from build123d import *

# Parameters (mm, degrees)
F1_DEPTH = 63.5
F0_W     = 25.4
F0_H     = 19.05
F2_DEPTH = 25.4
F3_DEPTH = 7.9375
F4_R     = 6.35


with BuildPart() as f1:
    # F0 (on Front) → F1 (new body, symmetric)
    with BuildSketch(Plane.XZ):
        Polygon((41.275, -9.525), (41.275, 9.525), (22.225, 9.525), (-41.275, 9.525), (-41.275, -9.525), align=None)
    extrude(amount=F1_DEPTH, both=True)

    # F0 (on Front) → F2 (join, symmetric)
    with BuildSketch(Plane.XZ):
        with BuildLine():
            Line((22.225, 9.525), (41.275, 9.525))
            Line((41.275, 9.525), (41.275, 27.0002))
            ThreePointArc((41.275, 27.0002), (45.9246798487, 38.2255201513), (57.15, 42.8752))
            Line((57.15, 42.8752), (60.325, 42.8752))
            Line((60.325, 42.8752), (60.325, 61.9252))
            Line((60.325, 61.9252), (57.15, 61.9252))
            add(Edge.make_bspline(
                [(54.22326899, 61.8023532465), (55.2121587279, 61.8549706116), (56.1881793337, 61.8959521575), (57.15, 61.9252)],
                knots=[108.6829517829, 108.6829517829, 108.6829517829, 108.6829517829, 111.5045361635, 111.5045361635, 111.5045361635, 111.5045361635], degree=3))
            ThreePointArc((54.22326899, 61.8023532465), (31.440354869, 50.6385115352), (22.225, 27.0002))
            Line((22.225, 27.0002), (22.225, 9.525))
        make_face()
        with Locations((73.025, 52.4002)):
            Rectangle(F0_W, F0_H)
    extrude(amount=F2_DEPTH, both=True)

    # F0 (on Front) → F3 (join, symmetric)
    with BuildSketch(Plane.XZ):
        with BuildLine():
            Line((-41.275, 9.525), (22.225, 9.525))
            Line((22.225, 9.525), (22.225, 27.0002))
            ThreePointArc((22.225, 27.0002), (31.440354869, 50.6385115352), (54.22326899, 61.8023532465))
            add(Edge.make_bspline(
                [(-41.275, 9.525), (-41.0511784846, 40.4851844974), (16.1328058977, 59.7756158605), (54.22326899, 61.8023532465)],
                knots=[0, 0, 0, 0, 108.6829517829, 108.6829517829, 108.6829517829, 108.6829517829], degree=3))
        make_face()
    extrude(amount=F3_DEPTH, both=True)

    # F4
    f4_edges = [f1.edges().sort_by_distance(p)[0] for p in [
        (41.275, -63.5, 0),
        (-41.275, -63.5, 0),
        (-41.275, 63.5, 0),
        (41.275, 63.5, 0),
    ]]
    fillet(f4_edges, radius=F4_R)


solid = f1.part
Geometry check sheet. Reference: the model listing, model coordinates, mm. A direction names the side the tool comes from. Give positions to 0.01 mm unless a question says otherwise; leave off trailing zeros. Loops run counter-clockwise (first coordinate to the right, second up) from the corner with the lowest first, then second, coordinate; pieces in that order, holes last. Notation, with made-up numbers: (58.25, 85.5) -> (108.25, 85.5) arc R31 cw to (108.25, 120.5) -> close; hole circle Ø9 at (-36, 42). An arc over 180 degrees is marked (long way). Answer in a Markdown table with one row per item. Add a question column.
1) Cross-section at A-A on z = 4.5. Record the boundary of the cut face in (x, y) (3 decimals).
2) Cross-section at B-B on y = 31. Record the boundary of the cut face in (x, z) (3 decimals).
3) Material ranges on probe 1 along Y at (x, z) = (39.5, 38.5); probe 2 along Z at (x, y) = (31, -45) (3 decimals); probe 3 along Z at (x, y) = (58, 24.5), recorded low to high. Write a range as from..to.
4) Gauge pin test, flat ends, axial feed: P1, Ø1, axis at y = -18, z = 3, coming from the +X side (3 decimals); P2, Ø5, axis at y = 16, z = 16, coming from the -X side (3 decimals); P3, Ø3, axis at x = 48, y = 5.5, coming from the +Z side; P4, Ø8, axis at x = -21, z = 10.5, coming from the +Y side. Record the tip position at first contact, or that the pin passes through.
5) Set-up check for faces 1 (the face through (31.688, 16.547, 50.905)), 2 (the face through (31.688, -16.791, 50.905)), 3 (the face through (41.275, -1, 4)): record each of +Z, -Z, +X, -X, +Y, -Y from which the full face is reachable in a straight line by a thin tool's end or side.
Outcome:
| question | item | result |
|---|---|---|
| 1 | outline | (-41.275, -57.15) arc R6.35 ccw to (-34.925, -63.5) -> (34.925, -63.5) arc R6.35 ccw to (41.275, -57.15) -> (41.275, 57.15) arc R6.35 ccw to (34.925, 63.5) -> (-34.925, 63.5) arc R6.35 ccw to (-41.275, 57.15) -> close |
| 2 | outline | (-41.275, -9.525) -> (41.275, -9.525) -> (41.275, 9.525) -> (-41.275, 9.525) -> close |
| 3 | probe 1 | y = -25.4..25.4 |
| 3 | probe 2 | z = -9.525..9.525 |
| 3 | probe 3 | z = 42.88..61.93 |
| 4 | P1 | stops at x = 41.275 |
| 4 | P2 | stops at x = 22.225 |
| 4 | P3 | stops at z = 61.47 |
| 4 | P4 | stops at y = 63.5 |
| 5 | face 1 | +Z, -X, +Y |
| 5 | face 2 | +Z, -X, -Y |
| 5 | face 3 | -Z, +X, +Y, -Y |
